```python
from build123d import *

# Parameters (mm, degrees)
F0_W     = 28.358727
F0_H     = 10.653684
F1_DEPTH = 0.5
F2_DEPTH = 2


with BuildPart() as f1:
    # F0 (on Top) → F1 (new body)
    with BuildSketch(Plane.XY):
        with Locations((0.097342, -0.292027)):
            Rectangle(F0_W, F0_H)
        Polygon((-12.437687, 4.361372), (-11.831026, 4.483848), (-11.000611, 4.483848), (-10.170197, 4.483848), (-9.339782, 4.483848), (-8.509368, 4.483848), (-7.902696, 4.361372), (-7.407652, 4.027382), (-7.073832, 3.532167), (-6.951535, 2.925676), (-6.951535, 2.536048), (-6.951535, 2.14642), (-6.951535, 1.756791), (-6.951535, 1.367163), (-6.990814, 1.035404), (-7.101741, 0.721563), (-7.274166, 0.433052), (-7.497909, 0.17795), (-8.335223, -0.679854), (-9.172527, -1.537487), (-10.009832, -2.395121), (-10.847136, -3.252925), (-9.873236, -3.252925), (-8.899336, -3.252925), (-7.925436, -3.252925), (-6.951535, -3.252925), (-6.951535, -3.649093), (-6.951535, -4.045441), (-6.951535, -4.441788), (-6.951535, -4.837956), (-8.509708, -4.837956), (-10.06788, -4.837956), (-11.626052, -4.837956), (-13.184214, -4.837956), (-13.184214, -4.465558), (-13.184214, -4.093329), (-13.184214, -3.72109), (-13.184214, -3.348692), (-12.114717, -2.248356), (-11.04522, -1.148029), (-9.975723, -0.047703), (-8.906226, 1.052633), (-8.842317, 1.123421), (-8.795299, 1.208348), (-8.76602, 1.300675), (-8.75602, 1.394373), (-8.75602, 1.654125), (-8.75602, 1.913707), (-8.75602, 2.173289), (-8.75602, 2.433041), (-8.792199, 2.615455), (-8.890896, 2.762901), (-9.038341, 2.861768), (-9.220406, 2.897766), (-9.73647, 2.897766), (-10.252354, 2.897766), (-10.768248, 2.897766), (-11.284303, 2.897766), (-11.400399, 2.873657), (-11.495996, 2.807509), (-11.561114, 2.707602), (-11.585053, 2.583236), (-11.585053, 2.231507), (-11.585053, 1.879778), (-11.585053, 1.528038), (-11.585053, 1.176309), (-12.036, 1.176309), (-12.486956, 1.176309), (-12.937902, 1.176309), (-13.388848, 1.176309), (-13.388848, 1.613646), (-13.388848, 2.050992), (-13.388848, 2.488329), (-13.388848, 2.925676), (-13.266552, 3.532167), (-12.932732, 4.027382), align=None, mode=Mode.SUBTRACT)
        Polygon((-4.492161, 4.361372), (-3.88515, 4.483848), (-2.962578, 4.483848), (-2.040186, 4.483848), (-1.117784, 4.483848), (-0.195223, 4.483848), (0.403689, 4.361372), (0.894774, 4.027382), (1.227044, 3.532167), (1.34917, 2.925676), (1.34917, 1.370953), (1.34917, -0.183779), (1.34917, -1.738501), (1.34917, -3.293224), (1.227044, -3.898165), (0.894774, -4.38873), (0.403689, -4.71773), (-0.195223, -4.837956), (-1.117784, -4.837956), (-2.040186, -4.837956), (-2.962578, -4.837956), (-3.88515, -4.837956), (-4.492161, -4.71773), (-4.987716, -4.38873), (-5.321535, -3.898165), (-5.444012, -3.293224), (-5.444012, -1.738501), (-5.444012, -0.183779), (-5.444012, 1.370953), (-5.444012, 2.925676), (-5.321535, 3.532167), (-4.987716, 4.027382), align=None, mode=Mode.SUBTRACT)
        Polygon((2.31067, 4.07372), (2.31067, 4.483848), (3.120586, 4.483848), (3.930501, 4.483848), (4.740416, 4.483848), (5.550341, 4.483848), (5.550341, 2.153309), (5.550341, -0.177059), (5.550341, -2.507428), (5.550341, -4.837956), (5.099215, -4.837956), (4.648099, -4.837956), (4.196973, -4.837956), (3.745856, -4.837956), (3.745856, -2.917725), (3.745856, -0.997314), (3.745856, 0.923097), (3.745856, 2.843338), (3.387057, 2.843338), (3.028258, 2.843338), (2.669459, 2.843338), (2.31067, 2.843338), (2.31067, 3.253466), (2.31067, 3.663593), align=None, mode=Mode.SUBTRACT)
        Polygon((6.986897, 4.056661), (6.986897, 4.483848), (8.616897, 4.483848), (10.246897, 4.483848), (11.876897, 4.483848), (13.506897, 4.483848), (13.506897, 4.125049), (13.506897, 3.76625), (13.506897, 3.407451), (13.506897, 3.048662), (12.604825, 1.077092), (11.702752, -0.894647), (10.80068, -2.866397), (9.898608, -4.837956), (9.355334, -4.837956), (8.812061, -4.837956), (8.268778, -4.837956), (7.725504, -4.837956), (7.759613, -4.831066), (7.793722, -4.824357), (7.827821, -4.817637), (7.86193, -4.810747), (8.743503, -2.914275), (9.625076, -1.017983), (10.506649, 0.878318), (11.388222, 2.77478), (10.287896, 2.77478), (9.187559, 2.77478), (8.087233, 2.77478), (6.986897, 2.77478), (6.986897, 3.201957), (6.986897, 3.629314), align=None, mode=Mode.SUBTRACT)
        Polygon((-3.639527, -1.44809), (-3.639527, -2.719291), (-3.601628, -2.901706), (-3.499481, -3.049151), (-3.351176, -3.148018), (-3.174451, -3.184017), (-2.610849, -3.184017), (-2.047246, -3.184017), (-1.483643, -3.184017), (-0.920051, -3.184017), (-0.737466, -3.148018), (-0.589671, -3.049151), (-0.490454, -2.901706), (-0.454285, -2.719291), (-0.454285, -1.44809), (-0.454285, -0.177059), (-0.454285, 1.093972), (-0.454285, 2.365173), (-0.490454, 2.541557), (-0.589671, 2.689693), (-0.737466, 2.79184), (-0.920051, 2.829899), (-1.483643, 2.829899), (-2.047246, 2.829899), (-2.610849, 2.829899), (-3.174451, 2.829899), (-3.351176, 2.79184), (-3.499481, 2.689693), (-3.601628, 2.541557), (-3.639527, 2.365173), (-3.639527, 1.093972), (-3.639527, -0.177059), align=None)
    extrude(amount=F1_DEPTH)

    # F0 (on Top) → F2 (join)
    with BuildSketch(Plane.XY):
        Polygon((-11.000611, 4.483848), (-11.831026, 4.483848), (-12.437687, 4.361372), (-12.932732, 4.027382), (-13.266552, 3.532167), (-13.388848, 2.925676), (-13.388848, 2.488329), (-13.388848, 2.050992), (-13.388848, 1.613646), (-13.388848, 1.176309), (-12.937902, 1.176309), (-12.486956, 1.176309), (-12.036, 1.176309), (-11.585053, 1.176309), (-11.585053, 1.528038), (-11.585053, 1.879778), (-11.585053, 2.231507), (-11.585053, 2.583236), (-11.561114, 2.707602), (-11.495996, 2.807509), (-11.400399, 2.873657), (-11.284303, 2.897766), (-10.768248, 2.897766), (-10.252354, 2.897766), (-9.73647, 2.897766), (-9.220406, 2.897766), (-9.038341, 2.861768), (-8.890896, 2.762901), (-8.792199, 2.615455), (-8.75602, 2.433041), (-8.75602, 2.173289), (-8.75602, 1.913707), (-8.75602, 1.654125), (-8.75602, 1.394373), (-8.76602, 1.300675), (-8.795299, 1.208348), (-8.842317, 1.123421), (-8.906226, 1.052633), (-9.975723, -0.047703), (-11.04522, -1.148029), (-12.114717, -2.248356), (-13.184214, -3.348692), (-13.184214, -3.72109), (-13.184214, -4.093329), (-13.184214, -4.465558), (-13.184214, -4.837956), (-11.626052, -4.837956), (-10.06788, -4.837956), (-8.509708, -4.837956), (-6.951535, -4.837956), (-6.951535, -4.441788), (-6.951535, -4.045441), (-6.951535, -3.649093), (-6.951535, -3.252925), (-7.925436, -3.252925), (-8.899336, -3.252925), (-9.873236, -3.252925), (-10.847136, -3.252925), (-10.009832, -2.395121), (-9.172527, -1.537487), (-8.335223, -0.679854), (-7.497909, 0.17795), (-7.274166, 0.433052), (-7.101741, 0.721563), (-6.990814, 1.035404), (-6.951535, 1.367163), (-6.951535, 1.756791), (-6.951535, 2.14642), (-6.951535, 2.536048), (-6.951535, 2.925676), (-7.073832, 3.532167), (-7.407652, 4.027382), (-7.902696, 4.361372), (-8.509368, 4.483848), (-9.339782, 4.483848), (-10.170197, 4.483848), align=None)
        Polygon((-2.962578, 4.483848), (-3.88515, 4.483848), (-4.492161, 4.361372), (-4.987716, 4.027382), (-5.321535, 3.532167), (-5.444012, 2.925676), (-5.444012, 1.370953), (-5.444012, -0.183779), (-5.444012, -1.738501), (-5.444012, -3.293224), (-5.321535, -3.898165), (-4.987716, -4.38873), (-4.492161, -4.71773), (-3.88515, -4.837956), (-2.962578, -4.837956), (-2.040186, -4.837956), (-1.117784, -4.837956), (-0.195223, -4.837956), (0.403689, -4.71773), (0.894774, -4.38873), (1.227044, -3.898165), (1.34917, -3.293224), (1.34917, -1.738501), (1.34917, -0.183779), (1.34917, 1.370953), (1.34917, 2.925676), (1.227044, 3.532167), (0.894774, 4.027382), (0.403689, 4.361372), (-0.195223, 4.483848), (-1.117784, 4.483848), (-2.040186, 4.483848), align=None)
        Polygon((-3.601628, -2.901706), (-3.639527, -2.719291), (-3.639527, -1.44809), (-3.639527, -0.177059), (-3.639527, 1.093972), (-3.639527, 2.365173), (-3.601628, 2.541557), (-3.499481, 2.689693), (-3.351176, 2.79184), (-3.174451, 2.829899), (-2.610849, 2.829899), (-2.047246, 2.829899), (-1.483643, 2.829899), (-0.920051, 2.829899), (-0.737466, 2.79184), (-0.589671, 2.689693), (-0.490454, 2.541557), (-0.454285, 2.365173), (-0.454285, 1.093972), (-0.454285, -0.177059), (-0.454285, -1.44809), (-0.454285, -2.719291), (-0.490454, -2.901706), (-0.589671, -3.049151), (-0.737466, -3.148018), (-0.920051, -3.184017), (-1.483643, -3.184017), (-2.047246, -3.184017), (-2.610849, -3.184017), (-3.174451, -3.184017), (-3.351176, -3.148018), (-3.499481, -3.049151), align=None, mode=Mode.SUBTRACT)
        Polygon((3.120586, 4.483848), (2.31067, 4.483848), (2.31067, 4.07372), (2.31067, 3.663593), (2.31067, 3.253466), (2.31067, 2.843338), (2.669459, 2.843338), (3.028258, 2.843338), (3.387057, 2.843338), (3.745856, 2.843338), (3.745856, 0.923097), (3.745856, -0.997314), (3.745856, -2.917725), (3.745856, -4.837956), (4.196973, -4.837956), (4.648099, -4.837956), (5.099215, -4.837956), (5.550341, -4.837956), (5.550341, -2.507428), (5.550341, -0.177059), (5.550341, 2.153309), (5.550341, 4.483848), (4.740416, 4.483848), (3.930501, 4.483848), align=None)
        Polygon((8.616897, 4.483848), (6.986897, 4.483848), (6.986897, 4.056661), (6.986897, 3.629314), (6.986897, 3.201957), (6.986897, 2.77478), (8.087233, 2.77478), (9.187559, 2.77478), (10.287896, 2.77478), (11.388222, 2.77478), (10.506649, 0.878318), (9.625076, -1.017983), (8.743503, -2.914275), (7.86193, -4.810747), (7.827821, -4.817637), (7.793722, -4.824357), (7.759613, -4.831066), (7.725504, -4.837956), (8.268778, -4.837956), (8.812061, -4.837956), (9.355334, -4.837956), (9.898608, -4.837956), (10.80068, -2.866397), (11.702752, -0.894647), (12.604825, 1.077092), (13.506897, 3.048662), (13.506897, 3.407451), (13.506897, 3.76625), (13.506897, 4.125049), (13.506897, 4.483848), (11.876897, 4.483848), (10.246897, 4.483848), align=None)
    extrude(amount=F2_DEPTH)


solid = f1.part
```
Design review of the part built by this model. Coordinates are the model's own, in mm. A direction names the side the tool comes from. Coordinates: 2 decimals unless noted, no trailing zeros. Loops run counter-clockwise (first coordinate to the right, second up) from the corner with the lowest first, then second, coordinate; pieces in that order, holes last.
Q1. We need section A-A on z = 0.8. State how many separate pieces and enclosed holes the cut face has, and give its area (3 significant figures).
Reported:
separate pieces: 4
enclosed holes: 1
area: 123 mm2
Q2. The part is to be moulded in two halves that separate along Y. For faces 1 (the face through (9, -4.838, 1)), 2 (the face through (6.987, 4, 1)), 3 (the face through (-3.64, 0, 1)), 4 (the face through (-2, 4.484, 1)), say which applies: +Y half, -Y half, draft (parallel to the pull), parting line (faces both ways), or undercut.
Reported:
face 1: -Y half
face 2: draft
face 3: undercut
face 4: +Y half
Q3. Tool access review of faces 5 (the face through (3.746, -1, 1)), 6 (the face through (-2, 0, 0.5)), 7 (the face through (-2, -4.838, 1)), 8 (the face through (-13.389, 2, 1)): name each direction out of +Z, -Z, +X, -X, +Y, -Y from which nothing blocks a thin tool from reaching the whole face with its end or side.
Reported:
face 5: +Z, -Y
face 6: +Z
face 7: +Z, +X, -X, -Y
face 8: +Z, -X, +Y, -Y
Q4. To check wall thickness, follow line 1 (X direction, y = -1, z = 1.85); line 2 (Y direction, x = -2, z = 1.35); line 3 (X direction, y = -4, z = 1.75). State the ranges of each line that lie inside material, in increasing order.
Reported:
line 1: x = -10.9 to -8.65, -5.44 to -3.64, -0.45 to 1.35, 3.75 to 5.55, 9.63 to 11.65
line 2: y = -4.84 to -3.18, 2.83 to 4.48
line 3: x = -13.18 to -6.95, -5.25 to 1.16, 3.75 to 5.55, 8.24 to 10.28
Q5. For pin 1 (0.8 mm diameter, centred on x = -2.5, z = 1, fed in from -Y); pin 2 (1.1 mm diameter, centred on x = 3, z = 1.5, fed in from -Y); pin 3 (0.8 mm diameter, centred on y = 2, z = 1, fed in from -X), all flat-tipped, find the tip position at first contact; note any pin that passes through.
Reported:
pin 1: stops at y = -4.84
pin 2: stops at y = 2.84
pin 3: stops at x = -13.39
Q6. We need section B-B on x = 4.25. State the section outline as (y, z) points, and give its area (3 significant figures).
Reported:
outline: (-5.62, 0) - (5.03, 0) - (5.03, 0.5) - (4.48, 0.5) - (4.48, 2) - (-4.84, 2) - (-4.84, 0.5) - (-5.62, 0.5) - close
area: 19.3 mm2
